Here's how the part is built. I have some questions about the finished solid (model axes, mm). Face numbers are marked on the shaded views. A direction names the side the tool comes from. Coordinates: 2 decimals unless noted, no trailing zeros. Loops run counter-clockwise (first coordinate to the right, second up) from the corner with the lowest first, then second, coordinate; pieces in that order, holes last. Notation, with made-up numbers: (-21, 48.5) -> (3, 48.5) arc R23 cw to (3, 56.5) -> close; hole circle Ø5 at (-25, 14.5). An arc over 180 degrees is marked (long way). Answer as a JSON object with one key per item and string values. Group by question number.
Q1. I want a section at B-B on z = -5. Write out the boundary of the cut face in (x, y), then the cut area to 3 significant figures.
Q2. I want a section at C-C on y = 15. Write out the boundary of the cut face in (x, z), then the cut area to 3 significant figures.
Q3. On a 3-axis mill with a long thin cutter (end or side, diameter ignored), from which of +Z, -Z, +X, -X, +Y, -Y can I reach the whole of each face in a straight line? I mean the marked faces 1, 2, 3 and 4. Say none if no direction works.
Q4. I need wall thicknesses on line 1 (Y direction, x = 3.5, z = -13.5); line 2 (Z direction, x = -12, y = 14.5); line 3 (Y direction, x = -0.5, z = -24.5). Which ranges of each line are inside material? Lowest first, please.
Q5. I want a section at D-D on z = -23.75. Write out the boundary of the cut face in (x, y), then the cut area to 3 significant figures.
Q6. I want a section at A-A on x = -11. Write out the boundary of the cut face in (y, z).
Q7. I'm going to push flat-ended pins straight in: pin 1 (10 mm diameter, centred on y = 8.5, z = -24, fed in from -X); pin 2 (3 mm diameter, centred on y = 8, z = -24.5, fed in from -X); pin 3 (18 mm diameter, centred on y = -10, z = -11, fed in from +X); pin 4 (11.5 mm diameter, centred on y = 6.5, z = -24.5, fed in from +X). Where does each tip first touch, or does it pass through?
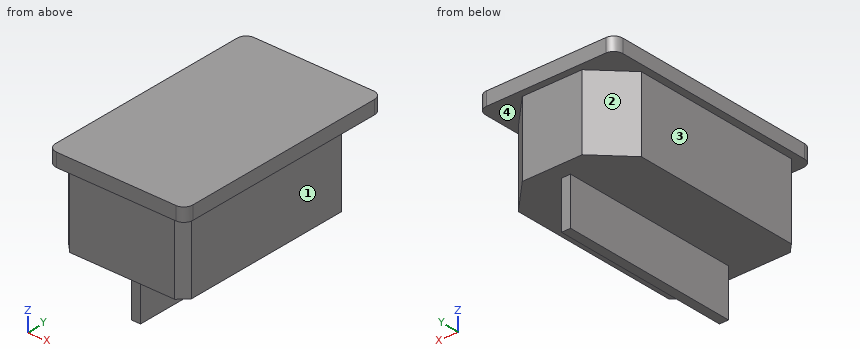
```python
from build123d import *

# Parameters (mm, degrees)
BOSS_EXTRUDE1_DEPTH = 3
BOSS_EXTRUDE2_DEPTH = 16.5
CHAMFER1_SIZE       = 2
SKETCH4_W           = 2
SKETCH4_H           = 40
BOSS_EXTRUDE3_DEPTH = 10.5


with BuildPart() as part:
    # Sketch1 → Boss-Extrude1 (new body)
    with BuildSketch(Plane.XY):
        with BuildLine():
            Line((-13.25, 25), (13.25, 25))
            ThreePointArc((13.25, 25), (14.664213562, 24.414213562), (15.25, 23))
            Line((15.25, 23), (15.25, -23))
            ThreePointArc((15.25, -23), (14.664213562, -24.414213562), (13.25, -25))
            Line((13.25, -25), (-13.25, -25))
            ThreePointArc((-13.25, -25), (-14.664213562, -24.414213562), (-15.25, -23))
            Line((-15.25, -23), (-15.25, 23))
            ThreePointArc((-15.25, 23), (-14.664213562, 24.414213562), (-13.25, 25))
        make_face()
    extrude(amount=-BOSS_EXTRUDE1_DEPTH)

    # Sketch2 → Boss-Extrude2 (add)
    with BuildSketch(Plane(origin=(0, 0, -3), x_dir=(-1, 0, 0), z_dir=(0, 0, -1))):
        Polygon((-13.65, 16.5), (-6.65, 23.5), (6.65, 23.5), (13.65, 16.5), (13.65, -23.5), (-13.65, -23.5), align=None)
    extrude(amount=BOSS_EXTRUDE2_DEPTH)

    # Chamfer1
    chamfer1_edges = [part.edges().sort_by_distance(p)[0] for p in [
        (-13.65, -23.5, -11.25),
        (13.65, -23.5, -11.25),
    ]]
    chamfer(chamfer1_edges, length=CHAMFER1_SIZE)

    # Sketch4 → Boss-Extrude3 (add)
    with BuildSketch(Plane(origin=(0, 0, -19.5), x_dir=(-1, 0, 0), z_dir=(0, 0, -1))):
        Rectangle(SKETCH4_W, SKETCH4_H)
    extrude(amount=BOSS_EXTRUDE3_DEPTH)


solid = part.part
```
Result set:
{
 "1": {"outline": "(-13.65, -21.5) -> (-11.65, -23.5) -> (11.65, -23.5) -> (13.65, -21.5) -> (13.65, 16.5) -> (6.65, 23.5) -> (-6.65, 23.5) -> (-13.65, 16.5) -> close", "area": "1,230 mm²"},
 "2": {"outline": "(-15.25, -3) -> (-13.65, -3) -> (-13.65, -19.5) -> (-1, -19.5) -> (-1, -30) -> (1, -30) -> (1, -19.5) -> (13.65, -19.5) -> (13.65, -3) -> (15.25, -3) -> (15.25, 0) -> (-15.25, 0) -> close", "area": "563 mm²"},
 "3": {"face 1": "-Z, +X, +Y, -Y", "face 2": "-Z, -X, +Y", "face 3": "-Z, -X, +Y, -Y", "face 4": "-Z"},
 "4": {"line 1": "y = -23.5 to 23.5", "line 2": "z = -19.5 to 0", "line 3": "y = -20 to 20"},
 "5": {"outline": "(-1, -20) -> (1, -20) -> (1, 20) -> (-1, 20) -> close", "area": "80.0 mm²"},
 "6": {"outline": "(-25, -3) -> (-23.5, -3) -> (-23.5, -19.5) -> (19.15, -19.5) -> (19.15, -3) -> (25, -3) -> (25, 0) -> (-25, 0) -> close"},
 "7": {"pin 1": "stops at x = -13.65", "pin 2": "stops at x = -1", "pin 3": "stops at x = 15.25", "pin 4": "stops at x = 13.65"}
}
